```python
from build123d import *

# Parameters (mm, degrees)
SKETCH_1_W               = 60
SKETCH_1_H               = 96
EXTRUDE_1_DEPTH          = 3
SKETCH_2_W               = 3
SKETCH_2_H               = 84
EXTRUDE_2_DEPTH          = 38
EXTRUDE_3_DEPTH          = 5
EXTRUDE_3_DEPTH_BACK     = 94.122011
SKETCH_4_R               = 7.35
SKETCH_5_R               = 3.95
EXTRUDE_4_DEPTH          = 8
FILLET_2_R               = 1
CUT_EXTRUDE_1_DEPTH      = 124.40908597
CUT_EXTRUDE_1_DEPTH_BACK = 124.40908597
SKETCH_9_R               = 1.5
FILLET_3_R               = 0.5
CUT_EXTRUDE_START        = 6
CUT_EXTRUDE_3_DEPTH      = 84
FILLET_6_R               = 3


# Read off the part's stored shape, not the designer's step: 切除-拉伸3
with BuildPart() as part:
    # 草图1 → 凸台-拉伸1 (new body)
    with BuildSketch(Plane.XY):
        with Locations((30, 48)):
            Rectangle(SKETCH_1_W, SKETCH_1_H)
    extrude(amount=EXTRUDE_1_DEPTH)

    # 草图2 → 凸台-拉伸2 (add)
    with BuildSketch(Plane(origin=(0, 0, 0), x_dir=(-1, 0, 0), z_dir=(0, 0, -1))):
        with Locations((-13.5, 48)):
            Rectangle(SKETCH_2_W, SKETCH_2_H)
    extrude(amount=EXTRUDE_2_DEPTH)

    # 草图4 → 凸台-拉伸3 (add, two sides: drawn at the far end of the back side and taken through both)
    with BuildSketch(Plane(origin=(0, 90, 0), x_dir=(1, 0, 0), z_dir=(0, 1, 0)).offset(-EXTRUDE_3_DEPTH_BACK)):
        with Locations(Location((15, 25, 0), (0, 0, 180))):
            Circle(SKETCH_4_R)
    extrude(amount=EXTRUDE_3_DEPTH + EXTRUDE_3_DEPTH_BACK)

    # 草图5 → 凸台-拉伸4 (add)
    with BuildSketch(Plane(origin=(0, 95, 0), x_dir=(1, 0, 0), z_dir=(0, 1, 0))):
        with Locations(Location((15, 25, 0), (0, 0, 270))):
            Circle(SKETCH_5_R)
    extrude(amount=EXTRUDE_4_DEPTH)

    # 圆角2
    fillet_2_edges = [part.edges().sort_by_distance(p)[0] for p in [
        (22.35, 95, -25),
        (15, 103, -28.95),
    ]]
    fillet(fillet_2_edges, radius=FILLET_2_R)

    # 草图9 → 切除-拉伸1 (cut, two sides: drawn at the far end of the back side and taken through both)
    with BuildSketch(Plane(origin=(0, 0, -28.95), x_dir=(-1, 0, 0), z_dir=(0, 0, -1)).offset(-CUT_EXTRUDE_1_DEPTH_BACK)):
        with Locations(Location((-15, 98.677988735, 0), (0, 0, 90.000000013))):
            Circle(SKETCH_9_R)
    extrude(amount=CUT_EXTRUDE_1_DEPTH + CUT_EXTRUDE_1_DEPTH_BACK, mode=Mode.SUBTRACT)

    # 圆角3
    fillet_3_edges = [part.edges().sort_by_distance(p)[0] for p in [
        (22.35, -4.122011, -25),
    ]]
    fillet(fillet_3_edges, radius=FILLET_3_R)

    # 切除-拉伸3 outline → 切除-拉伸3 (cut)
    with BuildSketch(Plane(origin=(0, 0, 0), x_dir=(1, 0, 0), z_dir=(0, 1, 0)).offset(CUT_EXTRUDE_START)):
        with BuildLine():
            Line((12, 38), (12, 31.709880774))
            ThreePointArc((12, 31.709880774), (13.466233996, 32.188189052), (15, 32.35))
            Line((15, 32.35), (15, 38))
            Line((15, 38), (12, 38))
        make_face()
    extrude(amount=CUT_EXTRUDE_3_DEPTH, mode=Mode.SUBTRACT)

    # 圆角6
    fillet_6_edges = [part.edges().sort_by_distance(p)[0] for p in [
        (12, 48, 0),
        (15, 48, 0),
    ]]
    fillet(fillet_6_edges, radius=FILLET_6_R)


solid = part.part
```
Source: CAD feature listing. Evaluate the final solid. Frame: model axes, mm. A direction names the side the tool comes from. Coordinates: 2 decimals unless noted, no trailing zeros. Write each loop counter-clockwise with the first axis right and the second up, starting at its lowest first coordinate (ties: lowest second). Pieces come first, ordered by that corner, then holes. Notation, with made-up numbers: (86.25, -24) - (130.25, -24) arc R19 ccw to (130.25, 4) - close; hole circle Ø8 at (6, 56). An arc over 180 degrees is marked (long way). Answer as a JSON object with one key per item and string values.
Q1. Draft query along Z for faces 1 (the flat face through (15, 103, -25)), 2 (the cylindrical face through (11.14, 48.59, -0.9)), 3 (the flat face through (14, 90, -8)), 4 (the flat face through (30, 49, 3)). Return one class per face: released by +Z, released by -Z, zero draft, split by the parting line, or undercut.
Ans:
{"face 1": "zero draft", "face 2": "undercut", "face 3": "undercut", "face 4": "released by +Z"}
Q2. First-contact query: pin 1 Ø4.5 at (y, z) = (65, -13.5) entering from +X; pin 2 Ø4.5 at (y, z) = (67.5, -7.5) entering from -X; pin 3 Ø1.5 at (x, z) = (28.5, 2) entering from -Y; pin 4 Ø12 at (x, z) = (27.5, -15.5) entering from +Y. Flat tips, straight axial feed; report the tip coordinate or a pass-through.
Ans:
{"pin 1": "stops at x = 15", "pin 2": "stops at x = 12", "pin 3": "stops at y = 0", "pin 4": "passes through"}
Q3. Set-up query: faces 5 (the flat face through (12, 47, -11)), 6 (the flat face through (30, 0, 1)), 7 (the flat face through (15, 47, -10)). Return all of +Z, -Z, +X, -X, +Y, -Y with unobstructed straight access to the full face (end or side cutting, diameter ignored); none if empty.
Ans:
{"face 5": "-X, +Y, -Y", "face 6": "+Z, +X, -X, -Y", "face 7": "+X, +Y, -Y"}
Q4. Section query A-A, the plane z = -25. Output: boundary loops of the cut face in (x, y).
Ans:
{"outline": "(7.65, -3.62) arc R0.5 ccw to (8.15, -4.12) - (21.85, -4.12) arc R0.5 ccw to (22.35, -3.62) - (22.35, 94) arc R1 ccw to (21.35, 95) - (18.95, 95) - (18.95, 102) arc R1 ccw to (17.95, 103) - (12.05, 103) arc R1 ccw to (11.05, 102) - (11.05, 95) - (8.65, 95) arc R1 ccw to (7.65, 94) - close; hole circle Ø3 at (15, 98.68)"}
Q5. Section query C-C, the plane z = -9. Output: boundary loops of the cut face in (x, y).
Ans:
{"outline": "(12, 6) - (15, 6) - (15, 90) - (12, 90) - close"}
Q6. Material intervals for line 1 (Z direction, x = 55, y = 34); line 2 (Z direction, x = 14, y = 93.5); line 3 (X direction, y = 65, z = -13), sorted ascending. Write a range as [from, to].
Ans:
{"line 1": "z = [0, 3]", "line 2": "z = [-32.28, -17.72], [0, 3]", "line 3": "x = [12, 15]"}
Q7. Section query B-B, the plane y = 35. Output: boundary loops of the cut face in (x, z).
Ans:
{"outline": "(0, 0) - (9, 0) arc R3 cw to (12, -3) - (12, -18.29) arc R7.35 ccw (long way) to (15, -17.65) - (15, -3) arc R3 cw to (18, 0) - (60, 0) - (60, 3) - (0, 3) - close"}
Q8. Section query D-D, the plane x = 30. Output: boundary loops of the cut face in (y, z), plus the area to 3 significant figures.
Ans:
{"outline": "(0, 0) - (96, 0) - (96, 3) - (0, 3) - close", "area": "288 mm2"}
